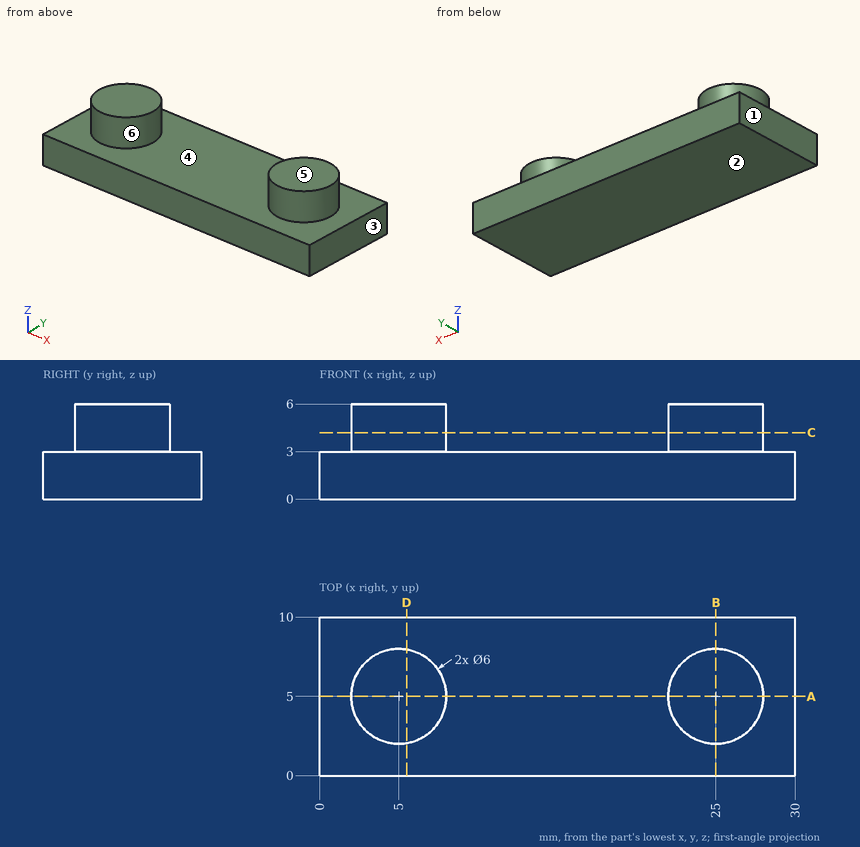
Geometry: see drawing. Coordinates: mm, zero at the bounding-box minimum. A direction names the side the tool comes from. Give positions to 0.01 mm unless a question says otherwise; leave off trailing zeros. Order: outer loops, then holes, each group sorted by start corner. A loop starts at its lowest first (then second) coordinate and runs counter-clockwise, first axis right, second up. Notation, with made-up numbers: (22, -20.5) - (70, -20.5) arc R20 ccw to (70, -2.5) - close; hole circle Ø1 at (46.5, 86). An arc over 180 degrees is marked (long way). Use a Markdown table: item, result.
(1) Line query: line 1 (X direction, y = 7, z = 4.75); line 2 (Z direction, x = 15, y = 8); line 3 (X direction, y = 3.75, z = 4.3). Output: solid intervals per line, ascending. Write a range as from..to.
Computed values:
| item | result |
|---|---|
| line 1 | x = 2.76..7.24, 22.76..27.24 |
| line 2 | z = 0..3 |
| line 3 | x = 2.27..7.73, 22.27..27.73 |
(2) Pin query (flat end, axial travel): pin 1 (1 mm diameter, centred on x = 24, z = 4.5, fed in from -Y); pin 2 (1 mm diameter, centred on x = 16, z = 4.5, fed in from +Y). Return the tip coordinate at first contact, or that it passes through.
Computed values:
| item | result |
|---|---|
| pin 1 | stops at y = 2.04 |
| pin 2 | passes through |
(3) Draft query along X for the marked faces 1, 2, 3 and 4. Return one class per face: released by +X, released by -X, zero draft, split by the parting line, or undercut.
Computed values:
| item | result |
|---|---|
| face 1 | released by -X |
| face 2 | zero draft |
| face 3 | released by +X |
| face 4 | undercut |
(4) Section query A-A (y = 5). Output: boundary loops of the cut face in (x, z).
Computed values:
| item | result |
|---|---|
| outline | (0, 0) - (30, 0) - (30, 3) - (28, 3) - (28, 6) - (22, 6) - (22, 3) - (8, 3) - (8, 6) - (2, 6) - (2, 3) - (0, 3) - close |
(5) Access query for the marked faces 5 and 6. Directions: +Z, -Z, +X, -X, +Y, -Y. A direction counts if a zero-diameter tool reaches every point of the face in a straight line with its end or side. Return the directions, or none.
Computed values:
| item | result |
|---|---|
| face 5 | +Z, +X, -X, +Y, -Y |
| face 6 | +Z |
(6) Section query D-D (x = 5.5). Output: boundary loops of the cut face in (y, z).
Computed values:
| item | result |
|---|---|
| outline | (0, 0) - (10, 0) - (10, 3) - (7.96, 3) - (7.96, 6) - (2.04, 6) - (2.04, 3) - (0, 3) - close |
(7) Section query C-C (z = 4.2). Output: boundary loops of the cut face in (x, y), then the cut area to 3 significant figures.
Computed values:
| item | result |
|---|---|
| outline | circle Ø6 at (5, 5); circle Ø6 at (25, 5) |
| area | 56.5 mm2 |
(8) Section query B-B (x = 25). Output: boundary loops of the cut face in (y, z).
Computed values:
| item | result |
|---|---|
| outline | (0, 0) - (10, 0) - (10, 3) - (8, 3) - (8, 6) - (2, 6) - (2, 3) - (0, 3) - close |
